Autodesk Inventor part; units mm, degrees
ref_plane "YZ Plane" through (0, 0, 0) normal (1, 0, 0) x (0, 1, 0)
ref_plane "XZ Plane" through (0, 0, 0) normal (0, 1, 0) x (-1, 0, 0)
ref_plane "XY Plane" through (0, 0, 0) normal (0, 0, 1) x (1, 0, 0)
sketch "Sketch1" plane through (0, 0, 0) normal (0, 0, 1) x (1, 0, 0)
  line L0 (34.3625, 20.8815) -> (-34.3625, 20.8815)
  line L1 (-34.3625, 20.8815) -> (-34.3625, -20.8815)
  line L2 (-34.3625, -20.8815) -> (34.3625, -20.8815)
  line L3 (34.3625, -20.8815) -> (34.3625, 20.8815)
  point P0 (0, 0)
extrude "Extrusion1" add sketch "Sketch1" along normal blind 2.5
sketch "Sketch2" plane through (0, 0, 2.5) normal (0, 0, 1) x (1, 0, 0)
  line L0 (0.2675, 5) -> (-4.7325, 5)
  line L1 (-4.7325, 5) -> (-4.7325, -5)
  line L2 (-4.7325, -5) -> (0.2675, -5)
  line L3 (0.2675, -5) -> (0.2675, 5)
  line L4 (28.7855, 5) -> (23.7855, 5)
  line L5 (23.7855, 5) -> (23.7855, -5)
  line L6 (23.7855, -5) -> (28.7855, -5)
  line L7 (28.7855, -5) -> (28.7855, 5)
  point P0 (0, 0)
  point P1 (-2.2325, 0)
  point P2 (26.2855, 0)
extrude "Extrusion2" cut sketch "Sketch2" against normal blind 2.5
properties part number "tail plate"
CAD build for the part. Positions are in the model's coordinates, mm. A direction names the side the tool comes from. Coordinates: 2 decimals unless noted, no trailing zeros. Loops run counter-clockwise (first coordinate to the right, second up) from the corner with the lowest first, then second, coordinate; pieces in that order, holes last. Notation, with made-up numbers: (-15, 13) - (-3, 13) arc R25 ccw to (-3, 31) - close; hole circle Ø10 at (37, 39). An arc over 180 degrees is marked (long way). Write item = value, one per line. Start each with the question number.
Q1. Pull direction Y, two halves, no side cores. Call faces 1 (the flat face through (-2, 5, 1)), 2 (the flat face through (-8, 0, 0)), 3 (the flat face through (0, -20.882, 1)), 4 (the flat face through (0, 20.882, 1)): pulls with the +Y half, pulls with the -Y half, needs draft (parallel to the pull), parting line crosses it, or undercut.
Q2. Cut at A-A, the plane y = 3.5. List the corners of the cut face in (x, z), then the cut area to 3 significant figures.
Q3. Drill centre lines: L1, parallel to X at y = 3, z = 2.25; L2, parallel to Y at x = 28, z = 0.95. Where is each one in solid material? Low to high.
Q4. Cut at B-B, the plane z = 0.8. List the corners of the cut face in (x, y), then the cut area to 3 significant figures.
Q5. Which spindle directions (+Z, -Z, +X, -X, +Y, -Y) get a long thin tool onto all of the face, cutting with end or side? Do faces 5 (the flat face through (-2, -5, 1)), 6 (the flat face through (-8, 0, 2.5)). Say none if no direction does.
Computed:
q1.face_1 = undercut
q1.face_2 = needs draft
q1.face_3 = pulls with the -Y half
q1.face_4 = pulls with the +Y half
q2.outline = (-34.36, 0) - (-4.73, 0) - (-4.73, 2.5) - (-34.36, 2.5) - close; (0.27, 0) - (23.79, 0) - (23.79, 2.5) - (0.27, 2.5) - close; (28.79, 0) - (34.36, 0) - (34.36, 2.5) - (28.79, 2.5) - close
q2.area = 147 mm²
q3.L1 = -34.36 to -4.73, 0.27 to 23.79, 28.79 to 34.36
q3.L2 = -20.88 to -5, 5 to 20.88
q4.outline = (-34.36, -20.88) - (34.36, -20.88) - (34.36, 20.88) - (-34.36, 20.88) - close; hole (-4.73, -5) - (0.27, -5) - (0.27, 5) - (-4.73, 5) - close; hole (23.79, -5) - (28.79, -5) - (28.79, 5) - (23.79, 5) - close
q4.area = 2,770 mm²
q5.face_5 = +Z, -Z
q5.face_6 = +Z, +X, -X, +Y, -Y
